Check sheet for the drawn part. Datum: minimum x, y, z corner. Units: mm. A direction names the side the tool comes from. Give positions to 0.01 mm unless a question says otherwise; leave off trailing zeros. Loops run counter-clockwise (first coordinate to the right, second up) from the corner with the lowest first, then second, coordinate; pieces in that order, holes last. Notation, with made-up numbers: (1.25, 83.5) - (24.25, 83.5) arc R21 ccw to (24.25, 118.5) - close; hole circle Ø5 at (10.25, 72). An arc over 180 degrees is marked (long way). One line per item, written item: value. Start each with the question number.
1. Scan lines: L1, parallel to Z at x = 12, y = 74; L2, parallel to Y at x = 22.75, z = 27.5; L3, parallel to Y at x = 6, z = 33.5 (1 decimal). Record each from-to range of solid material in increasing order. Write a range as [from, to].
2. Sectioned sample at A-A (z = 9.5). Record the cut outline in (x, y) (1 decimal).
3. Sectioned sample at D-D (x = 23.75). Count the separate pieces of the cut face and the enclosed holes in it, plus the area to 3 significant figures.
4. Mould release check, pull along X, two halves, no side actions. Record for the marked faces 1, 2, 3 and 4: pulls with the +X half, pulls with the -X half, needs draft (parallel to the pull), parting line crosses it, or undercut.
5. Access from +Z, -Z, +X, -X, +Y, -Y to the whole of each face (thin tool, end or side, straight path). Record for the marked faces 5, 6 and 7.
6. Gauge pin test, flat ends, axial feed: pin 1 (10 mm diameter, centred on y = 67, z = 17, fed in from -X); pin 2 (10 mm diameter, centred on y = 15.5, z = 18, fed in from +X); pin 3 (2.5 mm diameter, centred on x = 23, y = 29, fed in from -Z); pin 4 (12.5 mm diameter, centred on x = 14, z = 12.5, fed in from -Y) (1 decimal). Record the tip position at first contact, or that the pin passes through.
7. Sectioned sample at B-B (x = 17.75). Record the cut outline in (y, z) (1 decimal).
8. Sectioned sample at C-C (y = 14). Record the cut outline in (x, z).
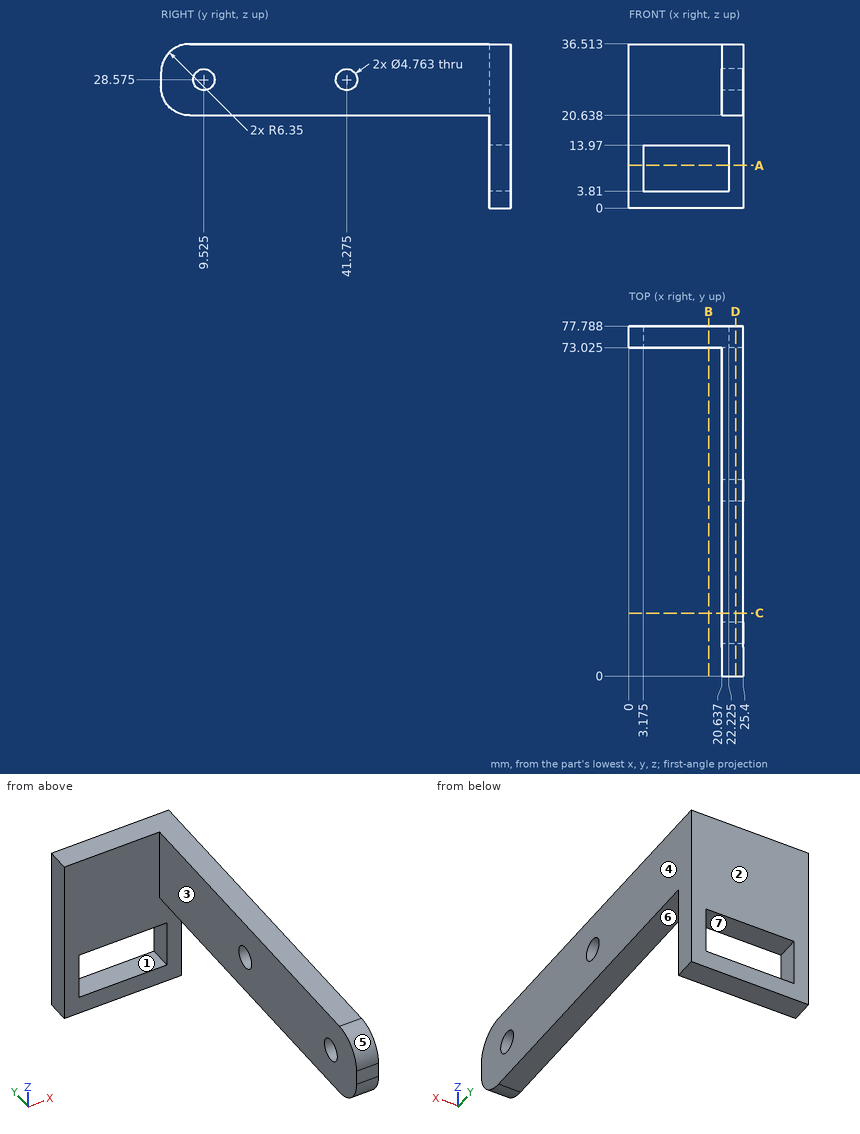
Results are:
1. L1: z = [0, 3.81], [13.97, 36.51]
1. L2: y = [0, 7.4], [11.65, 39.15], [43.4, 77.79]
1. L3: y = [73, 77.8]
2. outline: (0, 73) - (3.2, 73) - (3.2, 77.8) - (0, 77.8) - close; (22.2, 73) - (25.4, 73) - (25.4, 77.8) - (22.2, 77.8) - close
3. separate pieces: 1
3. enclosed holes: 2
3. area: 1,280 mm^2
4. face 1: undercut
4. face 2: needs draft
4. face 3: pulls with the -X half
4. face 4: pulls with the +X half
5. face 5: +Z, +X, -X, -Y
5. face 6: -Z, +X, -X, -Y
5. face 7: +Y, -Y
6. pin 1: stops at x = 20.64
6. pin 2: stops at x = 25.4
6. pin 3: stops at z = 20.64
6. pin 4: stops at y = 73
7. outline: (73, 0) - (77.8, 0) - (77.8, 3.8) - (73, 3.8) - close; (73, 14) - (77.8, 14) - (77.8, 36.5) - (73, 36.5) - close
8. outline: (20.64, 20.64) - (25.4, 20.64) - (25.4, 36.51) - (20.64, 36.51) - close
